The model under review builds one solid part; all positions refer to its coordinate system, in mm. Face numbers are marked on the shaded views. A direction names the side the tool comes from. Round coordinates to 2 decimals unless told otherwise and drop trailing zeros. Write each loop counter-clockwise with the first axis right and the second up, starting at its lowest first coordinate (ties: lowest second). Pieces come first, ordered by that corner, then holes. Notation, with made-up numbers: M 29.25,-29 L 52.25,-29 A19 cw 52.25,1 Z; hole C -2,54 d11. An arc over 180 degrees is marked long. One line per item, written item: value. Start each with the question number.
1) Take a section at C-C, the plane y = 7. Write out the cut boundary in (x, z).
2) Tool access review of the marked faces 1, 2 and 3: name each direction out of +Z, -Z, +X, -X, +Y, -Y from which nothing blocks a thin tool from reaching the whole face with its end or side.
3) Take a section at D-D, the plane x = 6. Write out the cut boundary in (y, z), and give its area (3 significant figures).
4) Wall thickness on probe 1 along Y at (x, z) = (6.75, 0); probe 2 along X at (y, z) = (-14, -2.5); probe 3 along Z at (x, y) = (-5.5, 12.6): over which ranges is each line inside the solid? List them lowest first.
5) Take a section at B-B, the plane z = 0. Write out the cut boundary in (x, y), and give its area (4 significant figures).
6) Take a section at A-A, the plane y = 12.6. Write out the cut boundary in (x, z), and give its area (3 significant figures).
7) For P1, Ø1, axis at x = -7.5, z = 1.5, coming from the +Y side; P2, Ø2.5, axis at y = 12.6, z = 0, coming from the +X side; P3, Ø2.5, axis at x = 0.5, z = -1.5, coming from the -Y side, all flat-tipped, find the tip position at first contact; note any pin that passes through.
8) Mouldability with a two-part tool opening along X and no side actions: class the marked faces 4, 5 and 6 as +X half, -X half, draft (parallel to the pull), parting line (faces both ways), or undercut.
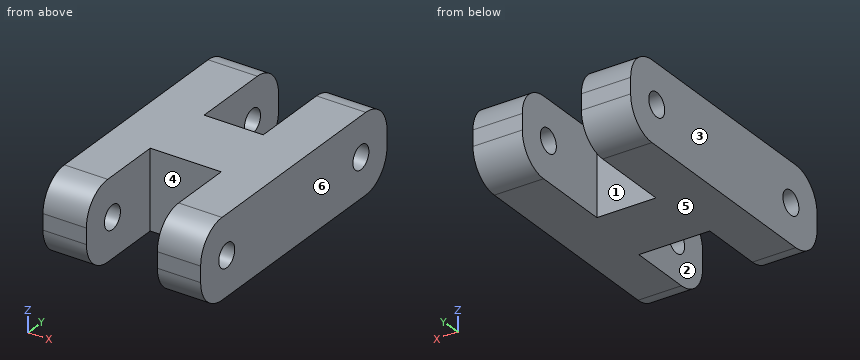
from build123d import *

# Parameters (mm, degrees)
CROQUIS1_R                 = 1.5
SALIENTE_EXTRUIR1_DEPTH    = 10
CORTAR_EXTRUIR1_DEPTH      = 21.766559657
CORTAR_EXTRUIR1_DEPTH_BACK = 21.766559657
CROQUIS2_W                 = 9
CROQUIS2_H                 = 12
CROQUIS2_W_2               = 7.5
CROQUIS2_H_2               = 14


with BuildPart() as part:
    # Croquis1 → Saliente-Extruir1 (new, symmetric)
    with BuildSketch(Plane(origin=(0, 0, 0), x_dir=(0, 0, -1), z_dir=(1, 0, 0))):
        with BuildLine():
            Line((-1, 17.5), (1, 17.5))
            ThreePointArc((1, 17.5), (3.828427125, 16.328427125), (5, 13.5))
            Line((5, 13.5), (5, -13.5))
            ThreePointArc((5, -13.5), (3.828427125, -16.328427125), (1, -17.5))
            Line((1, -17.5), (-1, -17.5))
            ThreePointArc((-1, -17.5), (-3.828427125, -16.328427125), (-5, -13.5))
            Line((-5, -13.5), (-5, 13.5))
            ThreePointArc((-5, 13.5), (-3.828427125, 16.328427125), (-1, 17.5))
        make_face()
        with Locations((0, 12.6)):
            Circle(CROQUIS1_R, mode=Mode.SUBTRACT)
        with Locations((0, -12.6)):
            Circle(CROQUIS1_R, mode=Mode.SUBTRACT)
    extrude(amount=SALIENTE_EXTRUIR1_DEPTH, both=True)

    # Croquis2 → Cortar-Extruir1 (cut, two sides: drawn at the far end of the back side and taken through both)
    with BuildSketch(Plane.XY.offset(-CORTAR_EXTRUIR1_DEPTH_BACK)):
        with Locations((0, -11.5)):
            Rectangle(CROQUIS2_W, CROQUIS2_H)
        with Locations((0, 10.5)):
            Rectangle(CROQUIS2_W_2, CROQUIS2_H_2)
    extrude(amount=CORTAR_EXTRUIR1_DEPTH + CORTAR_EXTRUIR1_DEPTH_BACK, mode=Mode.SUBTRACT)


solid = part.part
Checked values:
1. outline: M -10,-5 L -3.75,-5 L -3.75,5 L -10,5 Z; M 3.75,-5 L 10,-5 L 10,5 L 3.75,5 Z
2. face 1: +Z, -Z, +Y
2. face 2: +Z, -Z, -Y
2. face 3: +Z, -Z, -X, +Y, -Y
3. outline: M -17.5,-1 A4 ccw -13.5,-5 L 13.5,-5 A4 ccw 17.5,-1 L 17.5,1 A4 ccw 13.5,5 L -13.5,5 A4 ccw -17.5,1 Z; hole C -12.6,0 d3; hole C 12.6,0 d3
3. area: 322 mm2
4. probe 1: y = -17.5 to -14.1, -11.1 to 11.1, 14.1 to 17.5
4. probe 2: x = -10 to -4.5, 4.5 to 10
4. probe 3: z = -5 to -1.5, 1.5 to 5
5. outline: M -10,-17.5 L -4.5,-17.5 L -4.5,-14.1 L -10,-14.1 Z; M -10,-11.1 L -4.5,-11.1 L -4.5,-5.5 L 4.5,-5.5 L 4.5,-11.1 L 10,-11.1 L 10,11.1 L 3.75,11.1 L 3.75,3.5 L -3.75,3.5 L -3.75,11.1 L -10,11.1 Z; M -10,14.1 L -3.75,14.1 L -3.75,17.5 L -10,17.5 Z; M 3.75,14.1 L 10,14.1 L 10,17.5 L 3.75,17.5 Z; M 4.5,-17.5 L 10,-17.5 L 10,-14.1 L 4.5,-14.1 Z
5. area: 416.5 mm2
6. outline: M -10,-5 L -3.75,-5 L -3.75,-1.5 L -10,-1.5 Z; M -10,1.5 L -3.75,1.5 L -3.75,5 L -10,5 Z; M 3.75,-5 L 10,-5 L 10,-1.5 L 3.75,-1.5 Z; M 3.75,1.5 L 10,1.5 L 10,5 L 3.75,5 Z
6. area: 87.5 mm2
7. P1: stops at y = 17.5
7. P2: passes through
7. P3: stops at y = -5.5
8. face 4: undercut
8. face 5: draft
8. face 6: +X half
